```python
from build123d import *

# Parameters (mm, degrees)
F2_R     = 9.5
F3_DEPTH = 50
F5_DEPTH = 30


with BuildPart() as f1:
    # F0 (on Front) → F1 (revolve)
    with BuildSketch(Plane.XZ):
        Polygon((-28, 16), (-14.5, 11), (-14.5, -18), (0, -18), (0, 20), (-28, 20), align=None)
    revolve(axis=Axis((0, 0, 1), (0, 0, -1)))

    # F2 (on Top) → F3 (cut, symmetric)
    with BuildSketch(Plane.XY):
        Circle(F2_R)
    extrude(amount=F3_DEPTH, both=True, mode=Mode.SUBTRACT)

    # F4 (on Front) → F5 (cut)
    with BuildSketch(Plane.XZ):
        with BuildLine():
            ThreePointArc((3, 7.7993366867), (2.1213203436, 9.9206570303), (0, 10.7993366867))
            Line((0, 10.7993366867), (0, 4.7993366867))
            ThreePointArc((0, 4.7993366867), (2.1213203436, 5.6780163432), (3, 7.7993366867))
        make_face()
        with BuildLine():
            ThreePointArc((3, -8.1787835807), (2.1213203436, -6.0574632371), (0, -5.1787835807))
            ThreePointArc((0, -5.1787835807), (-2.1213203436, -10.3001039242), (3, -8.1787835807))
        make_face()
        with BuildLine():
            Line((0, 4.7993366867), (0, 10.7993366867))
            ThreePointArc((0, 10.7993366867), (-3, 7.7993366867), (0, 4.7993366867))
        make_face()
    extrude(amount=F5_DEPTH, mode=Mode.SUBTRACT)


solid = f1.part
```
Can you work these out from the model? Positions are in its coordinate system, mm. A direction names the side the tool comes from. Coordinates: 2 decimals unless noted, no trailing zeros. Loops run counter-clockwise (first coordinate to the right, second up) from the corner with the lowest first, then second, coordinate; pieces in that order, holes last. Notation, with made-up numbers: (61, 13.5) -> (91, 13.5) arc R7 cw to (91, 19.5) -> close; hole circle Ø8 at (45.25, 80). An arc over 180 degrees is marked (long way). Put each result on its own line as item: value. Start each with the question number.
Q1. I want a section at B-B (z = -14.5). Write out the boundary of the cut face in (x, y).
Q2. If I drill on line 1 (Y direction, x = 0, z = -1); line 2 (Y direction, x = 4, z = 4); line 3 (Z direction, x = 20, y = 14), over which ranges is the centre line in solid material (lowest first)? Write a range as [from, to].
Q3. I'm going to push flat-ended pins straight in: P1, Ø3.5, axis at x = 0, z = -8.18, coming from the -Y side; P2, Ø2, axis at x = -6.5, z = -4.5, coming from the +Y side. Where does each tip first touch, or does it pass through?
Q4. I want a section at A-A (y = 0). Write out the boundary of the cut face in (x, z).
Q5. Thinking about a two-plate mould opening in Y: for faces 1 (the face through (5.11, 8.01, 1.27)), 2 (the face through (3.285, -14.795, 11.243)), 3 (the face through (0, -12, 20)), which applies, pulls with the +Y half, pulls with the -Y half, needs draft (parallel to the pull), parting line crosses it, or undercut?
Q6. For faces 4 (the face through (-6.691, -12.864, -3.703)), 5 (the face through (-3, -9.5, -18)), which set-ups out of +Z, -Z, +X, -X, +Y, -Y let a thin tool reach every point of the face, with its end or its side?
Taken from the geometry:
1. outline: circle Ø29 at (0, 0); hole circle Ø19 at (0, 0)
2. line 1: y = [-14.5, -9.5], [9.5, 14.5]
2. line 2: y = [-13.94, -8.62], [8.62, 13.94]
2. line 3: z = [14.67, 20]
3. P1: stops at y = 9.34
3. P2: stops at y = 13.42
4. outline: (-28, 16) -> (-14.5, 11) -> (-14.5, -18) -> (-9.5, -18) -> (-9.5, 20) -> (-28, 20) -> close; (9.5, -18) -> (14.5, -18) -> (14.5, 11) -> (28, 16) -> (28, 20) -> (9.5, 20) -> close
5. face 1: undercut
5. face 2: parting line crosses it
5. face 3: needs draft
6. face 4: -Z
6. face 5: -Z, +X, -X, +Y, -Y
